Check sheet for the drawn part. Datum: minimum x, y, z corner. Units: mm. Coordinates: 2 decimals unless noted, no trailing zeros. Order: outer loops, then holes, each group sorted by start corner. A loop starts at its lowest first (then second) coordinate and runs counter-clockwise, first axis right, second up.
1. Draft check along X on the marked faces 1, 2 and 3. Enter one of: released by +X, released by -X, zero draft, split by the parting line, or undercut.
2. Cross-section at D-D (z = 1.5). Enter the section's corners in (x, y).
3. Cross-section at C-C (x = 2.5). Enter the section's corners in (y, z).
4. Thickness scan on line 1 (X direction, y = 1.6, z = 5) (1 decimal); line 2 (Z direction, x = 3.5, y = 4.4); line 3 (Z direction, x = 7, y = 1.9) (1 decimal). Record the ranges inside material, lowest first.
5. Cross-section at B-B (y = 4.75). Enter the section's corners in (x, z), then the cut area to 3 significant figures.
6. Cross-section at A-A (z = 4.5). Enter the section's corners in (x, y).
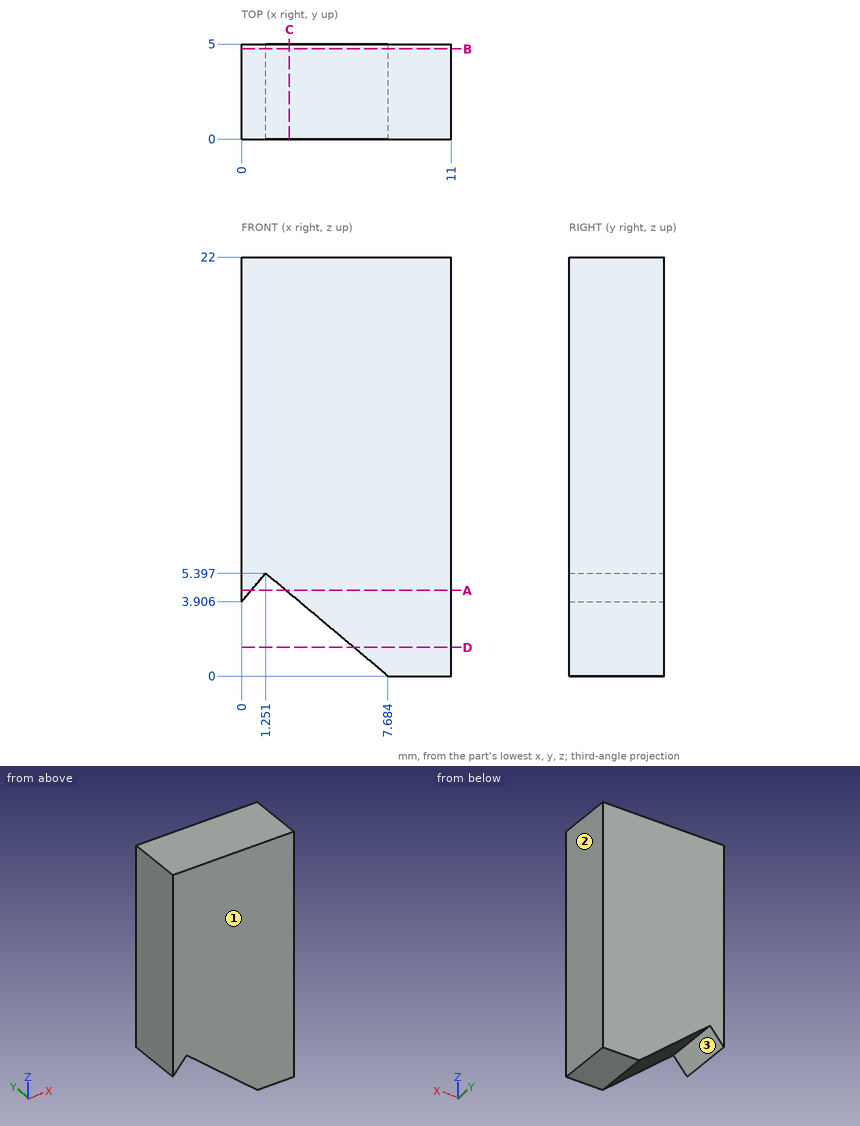
Data:
1. face 1: zero draft
1. face 2: released by +X
1. face 3: undercut
2. outline: (5.9, 0) - (11, 0) - (11, 5) - (5.9, 5) - close
3. outline: (0, 4.35) - (5, 4.35) - (5, 22) - (0, 22) - close
4. line 1: x = 0 to 0.9, 1.7 to 11
4. line 2: z = 3.51 to 22
4. line 3: z = 0.6 to 22
5. outline: (0, 3.91) - (1.25, 5.4) - (7.68, 0) - (11, 0) - (11, 22) - (0, 22) - close
5. area: 219 mm2
6. outline: (0, 0) - (0.5, 0) - (0.5, 5) - (0, 5) - close; (2.32, 0) - (11, 0) - (11, 5) - (2.32, 5) - close
